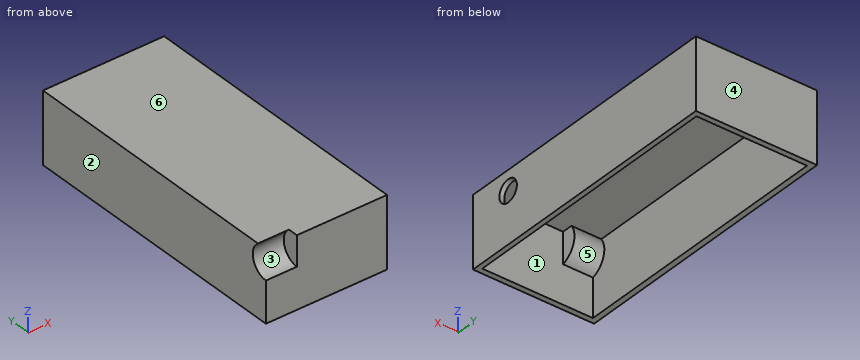
from build123d import *

# Parameters (mm, degrees)
SKETCH_W        = 54.7
SKETCH_H        = 127
PAD_DEPTH       = 32
SKETCH001_W     = 49.98
SKETCH001_H     = 121.98
POCKET_DEPTH    = 31.3
PAD001_DEPTH    = 16
SKETCH002_R     = 7.5
POCKET001_DEPTH = 14
SKETCH004_R     = 5
POCKET002_DEPTH = 5


with BuildPart() as part:
    # Sketch → Pad (new body)
    with BuildSketch(Plane.XY):
        with Locations((27.35, 63.5)):
            Rectangle(SKETCH_W, SKETCH_H)
    extrude(amount=PAD_DEPTH)

    # Sketch001 → Pocket (cut)
    with BuildSketch(Plane.XY):
        with Locations((27.5, 63.5)):
            Rectangle(SKETCH001_W, SKETCH001_H)
    extrude(amount=POCKET_DEPTH, mode=Mode.SUBTRACT)

    # Sketch003 → Pad001 (join)
    with BuildSketch(Plane.YZ):
        with BuildLine():
            ThreePointArc((0, 17), (8.215838, 22.325765), (6.708204, 32))
            Line((0, 32), (6.708204, 32))
            Line((0, 32), (0, 17))
        make_face()
    extrude(amount=PAD001_DEPTH)

    # Sketch002 → Pocket001 (cut)
    with BuildSketch(Plane.YZ):
        with Locations((0, 26)):
            Circle(SKETCH002_R)
    extrude(amount=POCKET001_DEPTH, mode=Mode.SUBTRACT)

    # Sketch004 (on DatumPlane) → Pocket002 (cut)
    with BuildSketch(Plane.YZ.offset(55)):
        with Locations((20.005968, 23)):
            Circle(SKETCH004_R)
    extrude(amount=-POCKET002_DEPTH, mode=Mode.SUBTRACT)


solid = part.part
Here's how the part is built. I have some questions about the finished solid (model axes, mm). Face numbers are marked on the shaded views. A direction names the side the tool comes from. Coordinates: 2 decimals unless noted, no trailing zeros. Order: outer loops, then holes, each group sorted by start corner. A loop starts at its lowest first (then second) coordinate and runs counter-clockwise, first axis right, second up.
Item 1: If we section it at B-B on y = 18.5: List the corners of the cut face in (x, z) for me.
Result sheet:
outline: (0, 0) - (2.51, 0) - (2.51, 31.3) - (52.49, 31.3) - (52.49, 27.77) - (54.7, 27.77) - (54.7, 32) - (0, 32) - close; (52.49, 0) - (54.7, 0) - (54.7, 18.23) - (52.49, 18.23) - close
Item 2: For P1, Ø25, axis at x = 38, y = 51, coming from the -Z side; P2, Ø9, axis at y = 20.01, z = 23, coming from the +X side; P3, Ø8, axis at y = 92, z = 6.5, coming from the -X side, each with a flat end and sliding along its axis, tell me the tip position at first contact or that it passes through.
Result sheet:
P1: stops at z = 31.3
P2: stops at x = 2.51
P3: stops at x = 0
Item 3: If we section it at C-C on x = 38: List the corners of the cut face in (y, z) for me.
Result sheet:
outline: (0, 0) - (2.51, 0) - (2.51, 31.3) - (124.49, 31.3) - (124.49, 0) - (127, 0) - (127, 32) - (0, 32) - close
Item 4: If we section it at D-D on y = 40.5: List the corners of the cut face in (x, z) for me.
Result sheet:
outline: (0, 0) - (2.51, 0) - (2.51, 31.3) - (52.49, 31.3) - (52.49, 0) - (54.7, 0) - (54.7, 32) - (0, 32) - close
Item 5: If we mould it in two halves opening along Z, with no side actions, what happens to the marked faces 3, 4, 5 and 6? For each: +Z half, -Z half, draft (parallel to the pull), parting line (faces both ways), or undercut.
Result sheet:
face 3: undercut
face 4: draft
face 5: undercut
face 6: +Z half
Item 6: If we section it at A-A on z = 9: List the corners of the cut face in (x, y) for me.
Result sheet:
outline: (0, 0) - (54.7, 0) - (54.7, 127) - (0, 127) - close; hole (2.51, 2.51) - (52.49, 2.51) - (52.49, 124.49) - (2.51, 124.49) - close
Item 7: For the marked faces 1 and 2, which set-ups out of +Z, -Z, +X, -X, +Y, -Y let a thin tool reach every point of the face, with its end or its side?
Result sheet:
face 1: -Z
face 2: +Z, -Z, -X, +Y, -Y
Item 8: I need wall thicknesses on line 1 (Y direction, x = 22.5, z = 6); line 2 (X direction, y = 19.5, z = 7); line 3 (Y direction, x = 6, z = 26.5). Which ranges of each line are inside material? Lowest first, please.
Result sheet:
line 1: y = 0 to 2.51, 124.49 to 127
line 2: x = 0 to 2.51, 52.49 to 54.7
line 3: y = 7.48 to 8.99, 124.49 to 127
